Geometry: final body of the model. Coordinates: model frame, mm. Coordinates: 2 decimals unless noted, no trailing zeros. Order: outer loops, then holes, each group sorted by start corner. A loop starts at its lowest first (then second) coordinate and runs counter-clockwise, first axis right, second up. Notation, with made-up numbers: M 89.25,27.25 L 137.25,27.25 A22 cw 137.25,62.25 Z; hole C 52.25,8 d5. An arc over 180 degrees is marked long. Write item = value, one per line.
from build123d import *

# Parameters (mm, degrees)
F1_DEPTH = 175
F2_W     = 3
F2_H     = 350
F3_DEPTH = 25
F5_DEPTH = 34.001
F7_DEPTH = 40


# Not quite as in the source:
# - a pattern or mirror of a feature is missing from the dataset's text; its kind, count and spacing are read off the source's solid


with BuildPart() as f1:
    # F0 (on Top) → F1 (new body, symmetric)
    with BuildSketch(Plane.XY):
        with BuildLine():
            ThreePointArc((20, 17), (19.1213203436, 19.1213203436), (17, 20))
            Line((17, 20), (-17, 20))
            ThreePointArc((-17, 20), (-19.1213203436, 19.1213203436), (-20, 17))
            Line((-20, 17), (-20, -17))
            ThreePointArc((-20, -17), (-19.1213203436, -19.1213203436), (-17, -20))
            Line((-17, -20), (17, -20))
            ThreePointArc((17, -20), (19.1213203436, -19.1213203436), (20, -17))
            Line((20, -17), (20, 17))
        make_face()
        with BuildLine():
            ThreePointArc((14, 17), (16.1213203436, 16.1213203436), (17, 14))
            Line((17, 14), (17, -14))
            ThreePointArc((17, -14), (16.1213203436, -16.1213203436), (14, -17))
            Line((14, -17), (-14, -17))
            ThreePointArc((-14, -17), (-16.1213203436, -16.1213203436), (-17, -14))
            Line((-17, -14), (-17, 14))
            ThreePointArc((-17, 14), (-16.1213203436, 16.1213203436), (-14, 17))
            Line((-14, 17), (14, 17))
        make_face(mode=Mode.SUBTRACT)
    extrude(amount=F1_DEPTH, both=True)

    # F2 (on face) → F3 (join)
    with BuildSketch(Plane.YZ.offset(20)):
        with Locations((-12.5, 0)):
            Rectangle(F2_W, F2_H)
    extrude(amount=F3_DEPTH)

    # F4 (on face) → F5 (cut, through all)
    with BuildSketch(Plane.XZ.offset(14)):
        Polygon((45, 175), (20, 175), (45, 150), align=None)
    f5 = extrude(amount=-F5_DEPTH, mode=Mode.SUBTRACT)

    # F5_copies: F5 across plane
    add(f5.mirror(Plane(origin=(0, 0, 0), x_dir=(-1, 0, 0), z_dir=(0, 0, -1))), mode=Mode.SUBTRACT)

    # F6 (on face) → F7 (join)
    with BuildSketch(Plane.XY.offset(175)):
        with BuildLine():
            Line((-20, 17), (-20, -17))
            ThreePointArc((-20, -17), (-19.1213203436, -19.1213203436), (-17, -20))
            Line((-17, -20), (17, -20))
            ThreePointArc((17, -20), (19.1213203436, -19.1213203436), (20, -17))
            Line((20, -17), (20, -14))
            Line((20, -14), (20, -11))
            Line((20, -11), (20, 17))
            ThreePointArc((20, 17), (19.1213203436, 19.1213203436), (17, 20))
            Line((17, 20), (-17, 20))
            ThreePointArc((-17, 20), (-19.1213203436, 19.1213203436), (-20, 17))
        make_face()
        with BuildLine():
            ThreePointArc((-14, -17), (-16.1213203436, -16.1213203436), (-17, -14))
            Line((-17, -14), (-17, 14))
            ThreePointArc((-17, 14), (-16.1213203436, 16.1213203436), (-14, 17))
            Line((-14, 17), (14, 17))
            ThreePointArc((14, 17), (16.1213203436, 16.1213203436), (17, 14))
            Line((17, 14), (17, -14))
            ThreePointArc((17, -14), (16.1213203436, -16.1213203436), (14, -17))
            Line((14, -17), (-14, -17))
        make_face(mode=Mode.SUBTRACT)
    f7 = extrude(amount=F7_DEPTH)

    # F7_copies: F7 across plane
    add(f7.mirror(Plane(origin=(0, 0, 0), x_dir=(-1, 0, 0), z_dir=(0, 0, -1))))


solid = f1.part
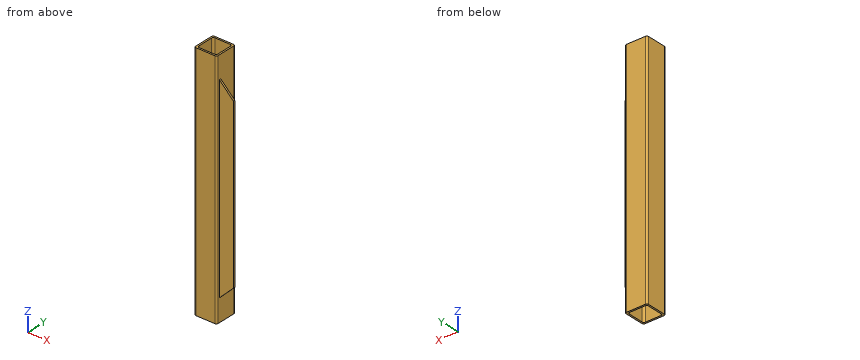
1) Pin query (flat end, axial travel): pin 1 (7.5 mm diameter, centred on x = 27.5, z = 16, fed in from +Y); pin 2 (6 mm diameter, centred on y = 1, z = 86, fed in from +X); pin 3 (6 mm diameter, centred on x = 21, z = 160.5, fed in from -Y). Return the tip coordinate at first contact, or that it passes through.
Numbers:
pin_1 = -11
pin_2 = 20
pin_3 = -19.83
2) Section A-A, the plane x = 5. Return loops of the section in (y, z), and give its area (3 significant figures).
Numbers:
outline = M -20,-215 L -17,-215 L -17,215 L -20,215 Z; M 17,-215 L 20,-215 L 20,215 L 17,215 Z
area = 2,580 mm²
3) Section D-D, the plane z = -187. Return loops of the section in (x, y), and give its area (3 significant figures).
Numbers:
outline = M -20,-17 A3 ccw -17,-20 L 17,-20 A3 ccw 20,-17 L 20,17 A3 ccw 17,20 L -17,20 A3 ccw -20,17 Z; hole M -17,-14 A3 ccw -14,-17 L 14,-17 A3 ccw 17,-14 L 17,14 A3 ccw 14,17 L -14,17 A3 ccw -17,14 Z
area = 444 mm²
4) Section C-C, the plane z = 15. Return loops of the section in (x, y).
Numbers:
outline = M -20,-17 A3 ccw -17,-20 L 17,-20 A3 ccw 20,-17 L 20,-14 L 45,-14 L 45,-11 L 20,-11 L 20,17 A3 ccw 17,20 L -17,20 A3 ccw -20,17 Z; hole M -17,-14 A3 ccw -14,-17 L 14,-17 A3 ccw 17,-14 L 17,14 A3 ccw 14,17 L -14,17 A3 ccw -17,14 Z
5) Line query: L1, parallel to X at y = 4, z = -105; L2, parallel to Y at x = 37, z = 3. Output: solid intervals per line, ascending.
Numbers:
L1 = -20 to -17, 17 to 20
L2 = -14 to -11
